Source: CAD feature listing. Evaluate the final solid. Frame: model axes, mm. Give positions to 0.01 mm unless a question says otherwise; leave off trailing zeros. Write each loop counter-clockwise with the first axis right and the second up, starting at its lowest first coordinate (ties: lowest second). Pieces come first, ordered by that corner, then holes. Notation, with made-up numbers: (14.5, 72.25) - (42.5, 72.25) arc R19 cw to (42.5, 87.25) - close; hole circle Ø2 at (49.25, 24). An arc over 180 degrees is marked (long way). Answer as a JSON object with one key per item and string values. Group by question number.
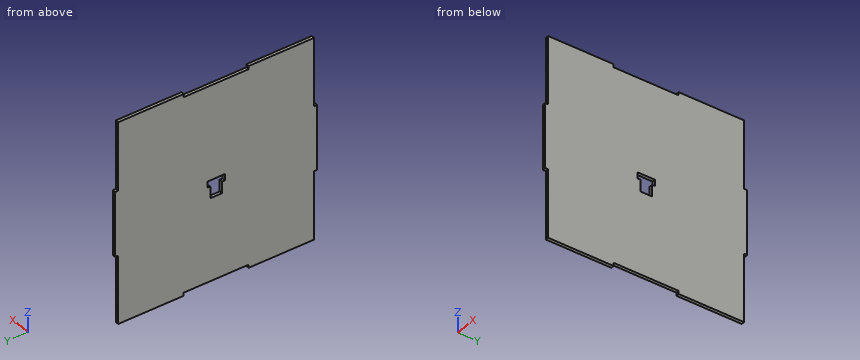
Autodesk Inventor part; units mm, degrees
ref_plane "YZ Plane" through (0, 0, 0) normal (1, 0, 0) x (0, 1, 0)
ref_plane "XZ Plane" through (0, 0, 0) normal (0, 1, 0) x (-1, 0, 0)
ref_plane "XY Plane" through (0, 0, 0) normal (0, 0, 1) x (1, 0, 0)
sketch "Esboço1" plane through (0, 0, 0) normal (1, 0, 0) x (0, 1, 0)
  line L0 (-129, 129) -> (129, 129)
  line L1 (129, 129) -> (129, -129)
  line L2 (129, -129) -> (-129, -129)
  line L3 (-129, -129) -> (-129, 129)
  line L4 (-129, 129) -> (129, -129) construction
  line L5 (129, 129) -> (-129, -129) construction
  point P0 (0, 0)
  dimension "d0" = 258
  dimension "d1" = 258
extrude "Extrusão1" add sketch "Esboço1" along normal mid plane 4
sketch "Esboço2" plane through (2, 0, 0) normal (1, 0, 0) x (0, 0, -1)
  line L0 (129, 129) -> (-129, 129)
  line L1 (-129, 129) -> (-41.5, 129)
  line L2 (-41.5, 129) -> (-41.5, 125)
  line L3 (-41.5, 125) -> (-129, 125)
  line L4 (-129, 125) -> (-129, 129)
  line L5 (129, 129) -> (41.5, 129)
  line L6 (41.5, 129) -> (41.5, 125)
  line L7 (41.5, 125) -> (129, 125)
  line L8 (129, 125) -> (129, 129)
  line L9 (-129, 129) -> (-129, -129)
  line L10 (-129, -129) -> (-41.5, -129)
  line L11 (-41.5, -129) -> (-41.5, -125)
  line L12 (-41.5, -125) -> (-129, -125)
  line L13 (-129, -125) -> (-129, -129)
  line L14 (129, -129) -> (129, 129)
  line L15 (129, -129) -> (41.5, -129)
  line L16 (41.5, -129) -> (41.5, -125)
  line L17 (41.5, -125) -> (129, -125)
  line L18 (129, -125) -> (129, -129)
  point P0 (0, 0)
  point P1 (129, -125)
  dimension "d4" = 87.5
  dimension "d5" = 4
  dimension "d6" = 87.5
  dimension "d7" = 4
  dimension "d8" = 83
  dimension "d9" = 87.5
  dimension "d10" = 4
  dimension "d11" = 87.5
  dimension "d12" = 4
  dimension "d13" = 83
extrude "Extrusão2" cut sketch "Esboço2" along normal through all both and the other way through all
sketch "Esboço3" plane through (2, 0, 0) normal (1, 0, 0) x (0, 0, -1)
  line L0 (-125, 41.5) -> (-133, 41.5)
  line L1 (-133, 41.5) -> (-133, -41.5)
  line L2 (-133, -41.5) -> (-125, -41.5)
  line L3 (-125, -41.5) -> (-125, 41.5)
  line L4 (-129, -125) -> (-129, 125)
  line L5 (-125, 41.5) -> (-133, -41.5) construction
  line L6 (-133, 41.5) -> (-125, -41.5) construction
  line L7 (125, -41.5) -> (133, -41.5)
  line L8 (133, -41.5) -> (133, 41.5)
  line L9 (133, 41.5) -> (125, 41.5)
  line L10 (125, 41.5) -> (125, -41.5)
  line L11 (129, 125) -> (129, -125)
  line L12 (125, -41.5) -> (133, 41.5) construction
  line L13 (133, -41.5) -> (125, 41.5) construction
  line L14 (-41.5, 125) -> (-129, 125)
  line L15 (-129, -125) -> (-41.5, -125)
  line L16 (129, 125) -> (41.5, 125)
  line L17 (41.5, -125) -> (129, -125)
  point P0 (0, 0)
  point P1 (-129, 0)
  point P2 (129, 0)
  dimension "d16" = 83
  dimension "d17" = 8
  dimension "d18" = 8
  dimension "d19" = 83
  dimension "d20" = 83.5
  dimension "d21" = 83.5
  dimension "d22" = 83.5
  dimension "d23" = 83.5
extrude "Extrusão3" cut sketch "Esboço3" along normal through all both and the other way through all
sketch "Esboço4" plane through (2, 0, 0) normal (1, 0, 0) x (0, 0, -1)
  line L0 (-4, -11) -> (4, -11)
  line L1 (4, -11) -> (4, 11)
  line L2 (4, 11) -> (-4, 11)
  line L3 (-4, 11) -> (-4, -11)
  line L4 (-4, -11) -> (4, 11) construction
  line L5 (4, -11) -> (-4, 11) construction
  point P0 (0, 0)
  dimension "d26" = 8
  dimension "d27" = 22
extrude "Extrusão4" cut sketch "Esboço4" against normal through all
sketch "Esboço5" plane through (2, 0, 0) normal (1, 0, 0) x (0, 0, -1)
  line L0 (4, 11) -> (4, 7.5)
  line L1 (4, -11) -> (4, 11)
  line L2 (4, 7.5) -> (19, 7.5)
  line L3 (19, 7.5) -> (19, -7.5)
  line L4 (19, -7.5) -> (4, -7.5)
  line L5 (4, -7.5) -> (4, 7.5)
  point P0 (0, 0)
  dimension "d30" = 3.5
  dimension "d32" = 15
extrude "Extrusão5" cut sketch "Esboço5" against normal through all
properties part number "TOPO POÇO"
Q1. Ray query, probe 1 along Z at (x, y) = (0.05, -3.5); probe 2 along Y at (x, z) = (-0.7, -17); probe 3 along Y at (x, z) = (-0.2, 64). Return the intervals inside material, ascending. Write a range as [from, to].
Q2. First-contact query: pin 1 Ø2 at (x, z) = (0.5, -127) entering from +Y; pin 2 Ø1.2 at (x, z) = (0, -127) entering from -Y; pin 3 Ø1.2 at (x, y) = (0, 3.5) entering from -Z. Flat tips, straight axial feed; report the tip coordinate or a pass-through.
Q3. Section B-B on z = -47. Return the cut outline in (x, y).
Q4. Section A-A on x = 0.2. Return the cut outline in (y, z).
Taken from the geometry:
{
 "1": {"probe 1": "z = [-125, -19], [4, 125]", "probe 2": "y = [-129, -7.5], [7.5, 129]", "probe 3": "y = [-125, 125]"},
 "2": {"pin 1": "stops at y = 125", "pin 2": "stops at y = -125", "pin 3": "stops at z = -125"},
 "3": {"outline": "(-2, -125) - (2, -125) - (2, 125) - (-2, 125) - close"},
 "4": {"outline": "(-129, -41.5) - (-125, -41.5) - (-125, -129) - (-41.5, -129) - (-41.5, -125) - (41.5, -125) - (41.5, -129) - (125, -129) - (125, -41.5) - (129, -41.5) - (129, 41.5) - (125, 41.5) - (125, 129) - (41.5, 129) - (41.5, 125) - (-41.5, 125) - (-41.5, 129) - (-125, 129) - (-125, 41.5) - (-129, 41.5) - close; hole (-11, -4) - (-7.5, -4) - (-7.5, -19) - (7.5, -19) - (7.5, -4) - (11, -4) - (11, 4) - (-11, 4) - close"}
}
